Job drawing, mm, ordinate dimensions from the low corner. One solid piece. Round coordinates to 2 decimals unless told otherwise and drop trailing zeros. Write each loop counter-clockwise with the first axis right and the second up, starting at its lowest first coordinate (ties: lowest second). Pieces come first, ordered by that corner, then holes.
1) Saw through at D-D on z = 21. Write the cut outline in (x, y).
2) Flat gauge pins, fed straight in: pin 1 (1 mm diameter, centred on y = 1, z = 20, fed in from +X); pin 2 (9 mm diameter, centred on x = 35.5, z = 35, fed in from +Y); pin 3 (0.6 mm diameter, centred on x = 54, y = 0.5, fed in from -Z); pin 4 (1 mm diameter, centred on x = 25.5, z = 32.5, fed in from -Y). Where does each tip first touch, or does it go through?
3) Pull direction Z, two halves, no side cores. Call the marked faces 1 and 2: +Z half, -Z half, draft (parallel to the pull), parting line (faces both ways), or undercut.
4) Drill centre lines: L1, parallel to X at y = 4.15, z = 35; L2, parallel to Z at x = 28.5, y = 1.2; L3, parallel to Y at x = 95, z = 45. Where is each one in solid material? Low to high.
5) Saw through at B-B on z = 35. Count the separate pieces of the cut face and the enclosed holes in it, and give its area (3 significant figures).
6) Saw through at A-A on x = 13.5. Write the cut outline in (y, z), and give its area (3 significant figures).
7) Saw through at C-C on y = 3.1. Write the cut outline in (x, z), and give its area (3 significant figures).
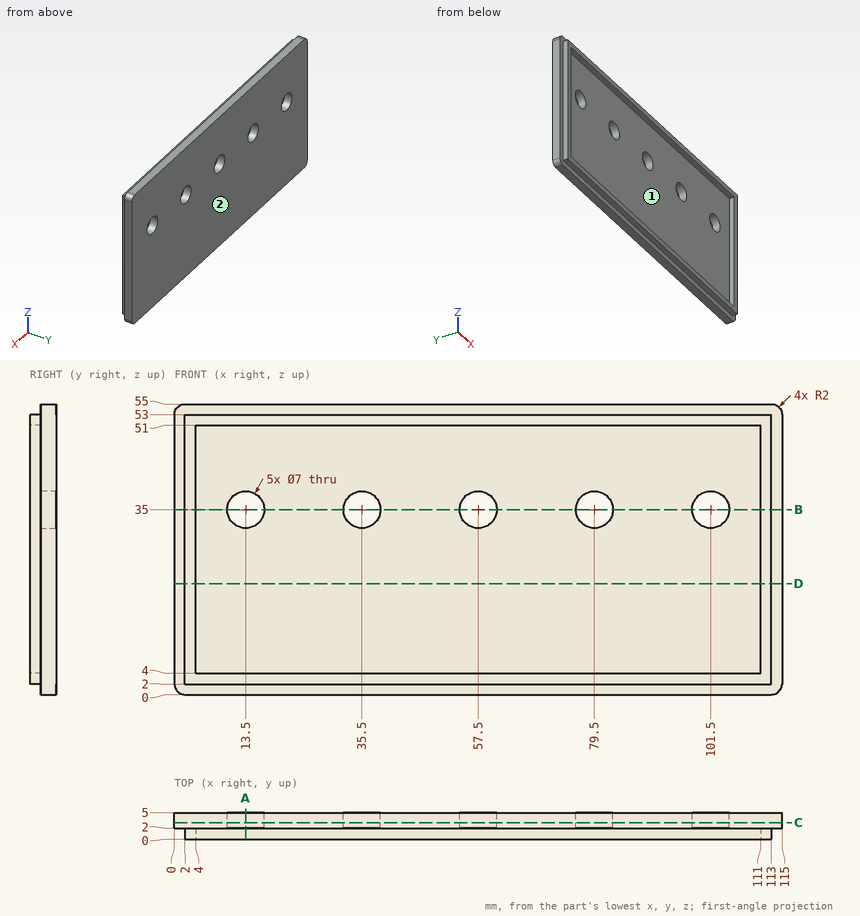
Completed:
1. outline: (0, 2) - (2, 2) - (2, 0) - (4, 0) - (4, 2) - (111, 2) - (111, 0) - (113, 0) - (113, 2) - (115, 2) - (115, 5) - (0, 5) - close
2. pin 1: stops at x = 113
2. pin 2: stops at y = 5
2. pin 3: stops at z = 2
2. pin 4: stops at y = 2
3. face 1: undercut
3. face 2: draft
4. L1: x = 0 to 10, 17 to 32, 39 to 54, 61 to 76, 83 to 98, 105 to 115
4. L2: z = 2 to 4, 51 to 53
4. L3: y = 2 to 5
5. separate pieces: 6
5. enclosed holes: 0
5. area: 248 mm2
6. outline: (0, 2) - (2, 2) - (2, 0) - (5, 0) - (5, 31.5) - (2, 31.5) - (2, 4) - (0, 4) - close; (0, 51) - (2, 51) - (2, 38.5) - (5, 38.5) - (5, 55) - (2, 55) - (2, 53) - (0, 53) - close
6. area: 152 mm2
7. outline: (0, 2) arc R2 ccw to (2, 0) - (113, 0) arc R2 ccw to (115, 2) - (115, 53) arc R2 ccw to (113, 55) - (2, 55) arc R2 ccw to (0, 53) - close; hole circle Ø7 at (13.5, 35); hole circle Ø7 at (35.5, 35); hole circle Ø7 at (57.5, 35); hole circle Ø7 at (79.5, 35); hole circle Ø7 at (101.5, 35)
7. area: 6,130 mm2
